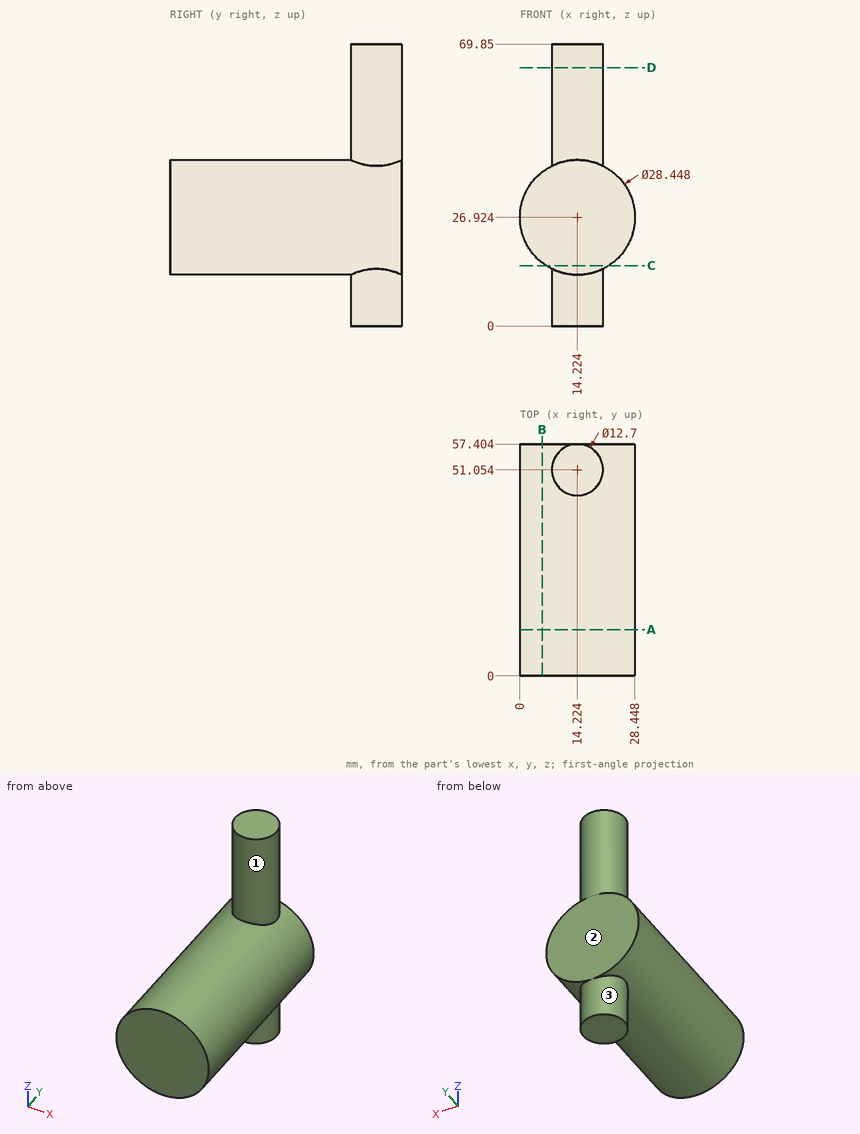
Verification items for this drawing (mm, ordinates from the low corner). A direction names the side the tool comes from. Give positions to 0.01 mm unless a question says otherwise; leave off trailing zeros. Order: outer loops, then holes, each group sorted by start corner. A loop starts at its lowest first (then second) coordinate and runs counter-clockwise, first axis right, second up. Notation, with made-up numbers: M -4.75,-24 L 47.25,-24 A28 cw 47.25,6 Z; hole C 50.25,-31 d2. An arc over 180 degrees is marked long. Use a Markdown table: item, result.
Item 1: Section check D-D (z = 64). Record the cut outline in (x, y), and give its area (3 significant figures).
Answers follow:
| item | result |
|---|---|
| outline | C 14.22,51.05 d12.7 |
| area | 127 mm2 |
Item 2: Material ranges on line 1 along Z through (x, y) = (14, 35.5); line 2 along Y through (x, z) = (14.5, 61); line 3 along Z through (x, y) = (6.25, 52), recorded low to high.
Answers follow:
| item | result |
|---|---|
| line 1 | z = 12.7 to 41.15 |
| line 2 | y = 44.71 to 57.4 |
| line 3 | z = 15.15 to 38.7 |
Item 3: Section check B-B (x = 5.5). Record the cut outline in (y, z).
Answers follow:
| item | result |
|---|---|
| outline | M 0,15.69 L 57.4,15.69 L 57.4,38.16 L 0,38.16 Z |
Item 4: Tool access check on the marked faces 1, 2 and 3. Record the directions out of +Z, -Z, +X, -X, +Y, -Y that give a thin tool (end or side, any length) a straight path to the whole face; none if there is none.
Answers follow:
| item | result |
|---|---|
| face 1 | +Z |
| face 2 | +Z, -Z, +X, -X, +Y |
| face 3 | -Z |
Item 5: Depth check by flat-ended pin: P1, Ø10, axis at y = 22, z = 49.5, coming from the -X side; P2, Ø2, axis at y = 35.5, z = 19.5, coming from the +X side; P3, Ø3, axis at y = 46.5, z = 35.5, coming from the -X side; P4, Ø10, axis at x = 14.5, y = 30, coming from the +Z side. Enter the tip coordinate at first touch or a pass-through.
Answers follow:
| item | result |
|---|---|
| P1 | passes through |
| P2 | stops at x = 26.91 |
| P3 | stops at x = 1.88 |
| P4 | stops at z = 41.15 |
Item 6: Section check C-C (z = 15). Record the cut outline in (x, y), and give its area (3 significant figures).
Answers follow:
| item | result |
|---|---|
| outline | M 6.47,0 L 21.98,0 L 21.98,57.4 L 6.47,57.4 Z |
| area | 890 mm2 |
Item 7: Section check A-A (y = 11.5). Record the cut outline in (x, z).
Answers follow:
| item | result |
|---|---|
| outline | C 14.22,26.92 d28.45 |
